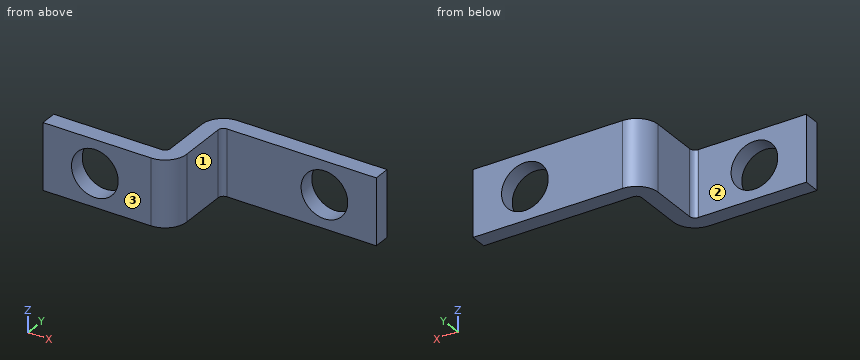
from build123d import *

# Parameters (mm, degrees)
SKETCH1_W                    = 25
SKETCH1_H                    = 12.7
BOSS_EXTRUDE1_DEPTH          = 3.175
EDGE_FLANGE1_STRIP_W         = 14.7
EDGE_FLANGE1_STRIP_H         = 3.175
EDGE_FLANGE1_STRIP_CUT_DEPTH = 12.7
EDGE_FLANGE1_DEPTH           = 12.7
EDGE_FLANGE2_STRIP_W         = 14.7
EDGE_FLANGE2_STRIP_H         = 3.175
EDGE_FLANGE2_STRIP_CUT_DEPTH = 12.7
EDGE_FLANGE2_DEPTH           = 12.7
M8_CLEARANCE_HOLE1_D         = 9


# Sheet-metal steps are written as plain solids
with BuildPart() as part:
    # Sketch1 → Boss-Extrude1 (new body)
    with BuildSketch(Plane(origin=(0, 0, 0), x_dir=(1, 0, 0), z_dir=(0, 1, 0))):
        with Locations((12.5, 6.35)):
            Rectangle(SKETCH1_W, SKETCH1_H)
    extrude(amount=BOSS_EXTRUDE1_DEPTH)

    # Edge-Flange1 strip (across the edge) → Edge-Flange1 strip cut (cut)
    with BuildSketch(Plane(origin=(25, 3.175, 0), x_dir=(-1, 0, 0), z_dir=(0, 0, -1))):
        with Locations((-3.175, -1.5875)):
            Rectangle(EDGE_FLANGE1_STRIP_W, EDGE_FLANGE1_STRIP_H)
    extrude(amount=EDGE_FLANGE1_STRIP_CUT_DEPTH, mode=Mode.SUBTRACT)

    # Edge-Flange1 section (across the edge) → Edge-Flange1 (add)
    with BuildSketch(Plane(origin=(25, 3.175, 0), x_dir=(-1, 0, 0), z_dir=(0, 0, -1))):
        with BuildLine():
            Line((0, 1), (0, 11.325))
            Line((0, 11.325), (3.175, 11.325))
            Line((3.175, 11.325), (3.175, 1))
            ThreePointArc((3.175, 1), (3.467893219, 0.292893219), (4.175, 0))
            Line((4.175, 0), (4.175, -3.175))
            ThreePointArc((4.175, -3.175), (1.222829189, -1.952170811), (0, 1))
        make_face()
    extrude(amount=EDGE_FLANGE1_DEPTH)

    # Edge-Flange2 strip (across the edge) → Edge-Flange2 strip cut (cut)
    with BuildSketch(Plane(origin=(25, 14.5, -12.7), x_dir=(0, -1, 0), z_dir=(0, 0, 1))):
        with Locations((-6.35, -1.5875)):
            Rectangle(EDGE_FLANGE2_STRIP_W, EDGE_FLANGE2_STRIP_H)
    extrude(amount=EDGE_FLANGE2_STRIP_CUT_DEPTH, mode=Mode.SUBTRACT)

    # Edge-Flange2 section (across the edge) → Edge-Flange2 (add)
    with BuildSketch(Plane(origin=(25, 14.5, -12.7), x_dir=(0, -1, 0), z_dir=(0, 0, 1))):
        with BuildLine():
            Line((-3.175, 1), (-3.175, 29.825))
            Line((-3.175, 29.825), (0, 29.825))
            Line((0, 29.825), (0, 1))
            ThreePointArc((0, 1), (0.292893219, 0.292893219), (1, 0))
            Line((1, 0), (1, -3.175))
            ThreePointArc((1, -3.175), (-1.952170811, -1.952170811), (-3.175, 1))
        make_face()
    extrude(amount=EDGE_FLANGE2_DEPTH)

    # M8 Clearance Hole1 (through all)
    with Locations(Plane(origin=(0, 17.675, 0), x_dir=(1, 0, 0), z_dir=(0, 1, 0))):
        with Locations((44.825, 6.35), (10, 6.35)):
            Hole(M8_CLEARANCE_HOLE1_D / 2)


solid = part.part
The listing builds one solid part. Answer for the finished solid, in the listing's coordinates (mm). Face numbers are marked on the shaded views. A direction names the side the tool comes from. Give positions to 0.01 mm unless a question says otherwise; leave off trailing zeros. Loops run counter-clockwise (first coordinate to the right, second up) from the corner with the lowest first, then second, coordinate; pieces in that order, holes last. Notation, with made-up numbers: M 75,47.25 L 132,47.25 A18 cw 132,60.25 Z; hole C 65.25,27.25 d6. An arc over 180 degrees is marked long. Answer as CSV lines item,"result".
Item 1: Which of the six approach directions +Z, -Z, +X, -X, +Y, -Y give full straight-line access (tool end or side, diameter ignored) to the marked faces 1, 2 and 3?
Values follow:
face 1,"+Z, -Z, +X, -Y"
face 2,"+Z, -Z, -X, +Y"
face 3,"+Z, -Z, +X, -X, -Y"
Item 2: The part is cut by section D-D (x = 51.5). Give the vertices of the cut face in (y, z) (3 decimals).
Values follow:
outline,"M 14.5,-12.7 L 17.675,-12.7 L 17.675,0 L 14.5,0 Z"
Item 3: The part is cut by section C-C (y = 1.75). Give the vertices of the cut face in (x, z).
Values follow:
outline,"M 0,-12.7 L 24.22,-12.7 L 24.22,0 L 0,0 Z; hole C 10,-6.35 d9"
Item 4: Given pin 1 Ø4 at (x, z) = (45, -4.5) entering from -Y; pin 2 Ø2 at (y, z) = (15.5, -7) entering from -X; pin 3 Ø4 at (x, z) = (46, -1.5) entering from -Y, each flat-ended and moving along its own axis, determine where each tip first touches the part or whether it passes through.
Values follow:
pin 1,"passes through"
pin 2,"stops at x = 21.95"
pin 3,"stops at y = 14.5"
Item 5: The part is cut by section A-A (x = 10). Give the vertices of the cut face in (y, z) (3 decimals), and give its area (3 significant figures).
Values follow:
outline,"M 0,-12.7 L 3.175,-12.7 L 3.175,-10.85 L 0,-10.85 Z; M 0,-1.85 L 3.175,-1.85 L 3.175,0 L 0,0 Z"
area,"11.7 mm^2"
Item 6: The part is cut by section B-B (z = -6.35). Give the vertices of the cut face in (x, y) (3 decimals), and give its area (3 significant figures).
Values follow:
outline,"M 0,0 L 5.5,0 L 5.5,3.175 L 0,3.175 Z; M 14.5,0 L 20.825,0 A4.175 ccw 25,4.175 L 25,13.5 A1 cw 26,14.5 L 40.325,14.5 L 40.325,17.675 L 26,17.675 A4.175 ccw 21.825,13.5 L 21.825,4.175 A1 cw 20.825,3.175 L 14.5,3.175 Z; M 49.325,14.5 L 54.825,14.5 L 54.825,17.675 L 49.325,17.675 Z"
area,"156 mm^2"
Item 7: Straight lines are drawn through the part: line 1 along Z through (x, y) = (10, 1.3); line 2 along X through (y, z) = (6.5, -7.75) (3 decimals); line 3 along Y through (x, z) = (34.5, -7.75) (3 decimals). For each, find the intervals that lie inside material, in ascending order. Write a range as [from, to].
Values follow:
line 1,"z = [-12.7, -10.85], [-1.85, 0]"
line 2,"x = [21.825, 25]"
line 3,"y = [14.5, 17.675]"
